CAD build for the part. Positions are in the model's coordinates, mm. Face numbers are marked on the shaded views. A direction names the side the tool comes from. Coordinates: 2 decimals unless noted, no trailing zeros. Write each loop counter-clockwise with the first axis right and the second up, starting at its lowest first coordinate (ties: lowest second). Pieces come first, ordered by that corner, then holes. Notation, with made-up numbers: (86.5, 26) -> (142.5, 26) arc R14 ccw to (142.5, 46) -> close; hole circle Ø8 at (84, 72.25). An arc over 180 degrees is marked (long way). Answer as CSV lines item,"result".
```python
from build123d import *

# Parameters (mm, degrees)
EXTRUDE_1_DEPTH     = 22
SKETCH_2_W          = 44
SKETCH_2_H          = 58
CUT_EXTRUDE_1_DEPTH = 7
FILLET_1_R          = 1
SKETCH_3_R          = 2
EXTRUDE_2_DEPTH     = 10


with BuildPart() as part:
    # Эскиз1 → Бобышка-Вытянуть1 (new, symmetric)
    with BuildSketch(Plane(origin=(0, 0, 0), x_dir=(0, 0, -1), z_dir=(1, 0, 0))):
        with BuildLine():
            Line((-49.5, 0), (0, 0))
            Line((0, 0), (0, -2.5))
            Line((0, -2.5), (-49.5, -2.5))
            ThreePointArc((-49.5, -2.5), (-51.974873734, -3.525126266), (-53, -6))
            Line((-53, -6), (-53, -3.5))
            ThreePointArc((-53, -3.5), (-51.974873734, -1.025126266), (-49.5, 0))
        make_face()
    extrude(amount=EXTRUDE_1_DEPTH, both=True)

    # Эскиз2 → Вырез-Вытянуть1 (cut)
    with BuildSketch(Plane(origin=(0, 0, 0), x_dir=(1, 0, 0), z_dir=(0, 1, 0))):
        with Locations((0, -29)):
            Rectangle(SKETCH_2_W, SKETCH_2_H)
        with BuildLine():
            Line((21.155172414, -33.5), (-21.155172414, -33.5))
            Line((-21.155172414, -33.5), (-21.720572868, -49.896613172))
            ThreePointArc((-21.720572868, -49.896613172), (-20.879918366, -52.084447111), (-18.72235487, -53))
            Line((-18.72235487, -53), (18.72235487, -53))
            ThreePointArc((18.72235487, -53), (20.879918366, -52.084447111), (21.720572868, -49.896613172))
            Line((21.720572868, -49.896613172), (21.155172414, -33.5))
        make_face(mode=Mode.SUBTRACT)
    extrude(amount=-CUT_EXTRUDE_1_DEPTH, mode=Mode.SUBTRACT)

    # Скругление1
    fillet_1_edges = [part.edges().sort_by_distance(p)[0] for p in [
        (0, -2.5, 33.5),
    ]]
    fillet(fillet_1_edges, radius=FILLET_1_R)

    # Эскиз3 → Бобышка-Вытянуть2 (add, symmetric)
    with BuildSketch(Plane(origin=(0, 0, 0), x_dir=(0, 0, -1), z_dir=(1, 0, 0))):
        with BuildLine():
            Line((-47, -8), (-47, -2.5))
            Line((-47, -2.5), (-41, -2.5))
            Line((-41, -2.5), (-41, -8))
            ThreePointArc((-41, -8), (-44, -11), (-47, -8))
        make_face()
        with Locations((-44, -8)):
            Circle(SKETCH_3_R, mode=Mode.SUBTRACT)
    extrude(amount=EXTRUDE_2_DEPTH, both=True)


solid = part.part
```
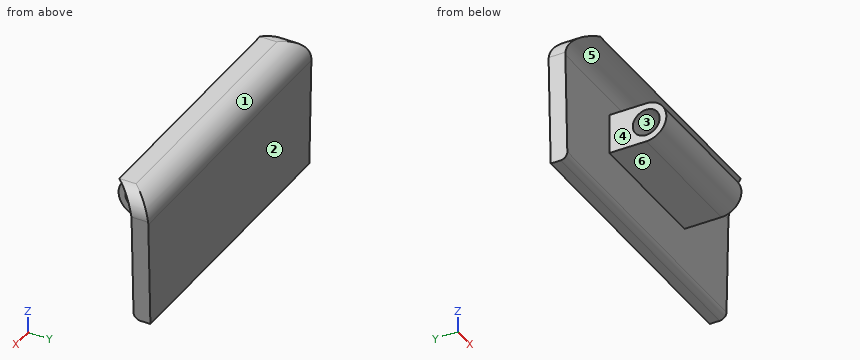
Item 1: Flat gauge pins, fed straight in: pin 1 (5 mm diameter, centred on y = -8.5, z = 48, fed in from +X); pin 2 (4 mm diameter, centred on y = -1, z = 38, fed in from +X); pin 3 (1.5 mm diameter, centred on y = -2.5, z = 48, fed in from +X). Where does each tip first touch, or does it go through?
Answer below:
pin 1,"stops at x = 10"
pin 2,"stops at x = 21.38"
pin 3,"stops at x = 21.68"
Item 2: Wall check: line 1 (Y direction, x = 2.75, z = 44); line 2 (Y direction, x = -6, z = 49.75); line 3 (Z direction, x = 4, y = -7.25). Give the ranges that are in metal, low to high. Write a range as from..to.
Answer below:
line 1,"y = -11..-10, -6..0"
line 2,"y = -2.51..-0.01"
line 3,"z = 41..42.15, 45.85..47"
Item 3: Two-plate mould, pull along Z, no slides. Class the marked faces 1, 2 and 3: pulls with the +Z half, pulls with the -Z half, needs draft (parallel to the pull), parting line crosses it, or undercut.
Answer below:
face 1,"pulls with the +Z half"
face 2,"needs draft"
face 3,"undercut"
Item 4: Saw through at B-B on y = -9. Give the cut face in (x, z).
Answer below:
outline,"(-10, 41.17) -> (10, 41.17) -> (10, 42.27) -> (-10, 42.27) -> close; (-10, 45.73) -> (10, 45.73) -> (10, 46.83) -> (-10, 46.83) -> close"
Item 5: Saw through at C-C on z = 44. Give the cut face in (x, y), and give its area (3 significant figures).
Answer below:
outline,"(-21.52, -2.5) -> (-10, -2.5) -> (-10, -6) -> (10, -6) -> (10, -2.5) -> (21.52, -2.5) -> (21.52, 0) -> (-21.52, 0) -> close; (-10, -11) -> (10, -11) -> (10, -10) -> (-10, -10) -> close"
area,"198 mm2"
Item 6: 3-axis set-ups, long thin cutter, end or side, ignore diameter. For the marked faces 4, 5 and 6: which of +Z, -Z, +X, -X, +Y, -Y reach the whole face in a straight line?
Answer below:
face 4,"-Z, -X, -Y"
face 5,"+X, -X, -Y"
face 6,"-Z, +X, -X, -Y"
Item 7: Saw through at A-A on x = -1.5. Give the cut face in (y, z).
Answer below:
outline,"(-8, 41) -> (-2.5, 41) -> (-2.5, 34.5) arc R1 ccw to (-1.5, 33.5) -> (0, 33.5) -> (0, 49.5) arc R3.5 ccw to (-3.5, 53) -> (-6, 53) arc R3.5 cw to (-2.5, 49.5) -> (-2.5, 47) -> (-8, 47) arc R3 ccw to start; hole circle Ø4 at (-8, 44)"
Item 8: Saw through at D-D on x = -11. Give the cut face in (y, z).
Answer below:
outline,"(-6, 53) arc R3.5 cw to (-2.5, 49.5) -> (-2.5, 34.5) arc R1 ccw to (-1.5, 33.5) -> (0, 33.5) -> (0, 49.5) arc R3.5 ccw to (-3.5, 53) -> close"
